Answer from the drawing. Dimensions are ordinates in mm from the lowest x, y and z of the part. Coordinates: 2 decimals unless noted, no trailing zeros. Write each loop counter-clockwise with the first axis right and the second up, starting at its lowest first coordinate (ties: lowest second). Pieces come first, ordered by that corner, then holes.
(1) Given pin 1 (4 mm diameter, centred on x = 44.5, y = 16, fed in from +Z); pin 2 (1 mm diameter, centred on x = 109, z = 134.5, fed in from -Y); pin 3 (8 mm diameter, centred on x = 17.5, y = 17, fed in from +Z), each flat-ended and moving along its own axis, determine where each tip first touches the part or whether it passes through.
(2) Find the intervals of material crossed by probe 1 along Z at (x, y) = (69, 1); probe 2 along Z at (x, y) = (67, 10.5); probe 3 along X at (y, z) = (23.25, 267), in increasing order.
(3) Section A-A on z = 250 is taken. Write down the section's boundary in (x, y).
(4) Section C-C on y = 7.5 is taken. Write down the section's boundary in (x, z), then the cut area to 3 significant figures.
(5) Section B-B on x = 75 is taken. Write down the section's boundary in (y, z), then the cut area to 3 significant figures.
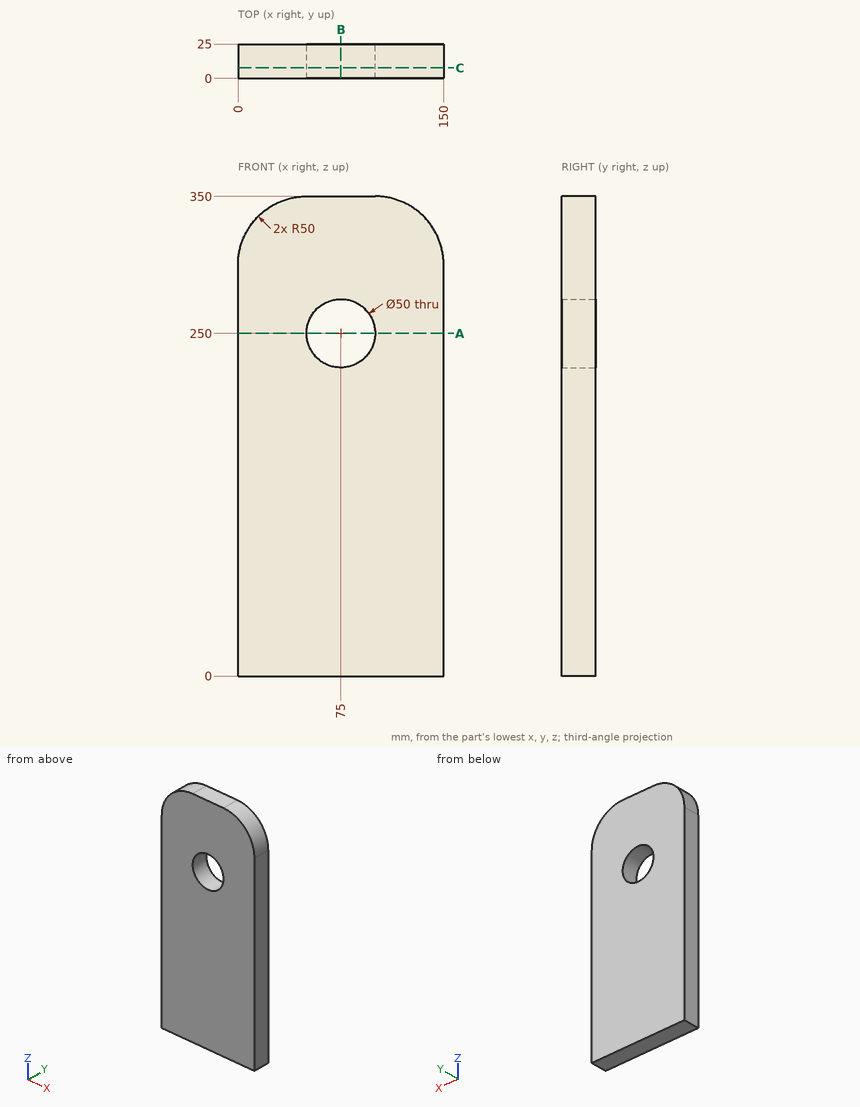
Response:
1. pin 1: stops at z = 349.88
1. pin 2: stops at y = 0
1. pin 3: stops at z = 341.08
2. probe 1: z = 0 to 225.73, 274.27 to 350
2. probe 2: z = 0 to 226.31, 273.69 to 350
2. probe 3: x = 0 to 56.67, 93.33 to 150
3. outline: (0, 0) - (50, 0) - (50, 25) - (0, 25) - close; (100, 0) - (150, 0) - (150, 25) - (100, 25) - close
4. outline: (0, 0) - (150, 0) - (150, 300) arc R50 ccw to (100, 350) - (50, 350) arc R50 ccw to (0, 300) - close; hole circle Ø50 at (75, 250)
4. area: 49,500 mm2
5. outline: (0, 0) - (25, 0) - (25, 225) - (0, 225) - close; (0, 275) - (25, 275) - (25, 350) - (0, 350) - close
5. area: 7,500 mm2
